```python
from build123d import *

# Parameters (mm, degrees)
F0_W            = 60
F0_H            = 55
F1_DEPTH        = 55
F2_T            = -3.5
F4_DEPTH        = 5
F6_D            = 3
F6_DEPTH        = 12
F6_TIP          = 0.9012909285
F8_D            = 3
F8_DEPTH        = 12
F8_TIP          = 0.9012909285
F7_W            = 41
F7_H            = 35
F9_DEPTH        = 25
F10_R           = 5
F11_DEPTH       = 7
F13_D           = 3
F13_DEPTH       = 5
F13_TIP         = 0.9012909285
F14_W           = 7
F14_H           = 3
F15_DEPTH       = 5
F16_W           = 7
F16_H           = 5
F17_DEPTH       = 5
F18_W           = 24
F18_H           = 6
F19_DEPTH       = 4
F21_D           = 3
F21_DEPTH       = 5
F21_TIP         = 0.9012909285
F23_D           = 3
F23_DEPTH       = 5
F23_TIP         = 0.9012909285
F24_W           = 10
F24_H           = 3
F25_DEPTH       = 10
F27_D           = 3.3
F27_DEPTH       = 5
F27_CSINK_D     = 6.72
F27_CSINK_ANGLE = 90
F27_TIP         = 0.9914200214
F29_D           = 3.3
F29_DEPTH       = 5
F29_CSINK_D     = 6.72
F29_CSINK_ANGLE = 90
F29_TIP         = 0.9914200214
F30_W           = 10
F30_H           = 3
F31_DEPTH       = 10
F32_DEPTH       = 10
F34_D           = 3.3
F34_DEPTH       = 5
F34_CSINK_D     = 6.72
F34_CSINK_ANGLE = 90
F34_TIP         = 0.9914200214


with BuildPart() as f1:
    # F0 (on Top) → F1 (new body)
    with BuildSketch(Plane.XY):
        Rectangle(F0_W, F0_H)
    extrude(amount=F1_DEPTH)

    # F2
    f2_openings = [f1.faces().sort_by_distance(p)[0] for p in [
        (0, 0, 55),
    ]]
    offset(amount=F2_T, openings=f2_openings)

    # F3 (on face) → F4 (cut)
    with BuildSketch(Plane.XZ.offset(27.5)):
        Polygon((19.05, 39.8), (-19.05, 39.8), (-19.05, 15.2), (0, 15.2), (19.05, 15.2), align=None)
    extrude(amount=-F4_DEPTH, mode=Mode.SUBTRACT)

    # F6
    with Locations(Plane.XZ.offset(27.5)):
        with Locations((-21.8598913223, 37.825), (-21.8598913223, 17.175), (21.5401086777, 17.175), (21.5401086777, 37.825)):
            Hole(F6_D / 2, depth=F6_DEPTH)
            with Locations((0, 0, -(F6_DEPTH + F6_TIP / 2))):  # 118° drill point
                Cone(0, F6_D / 2, F6_TIP, mode=Mode.SUBTRACT)

    # F8
    with Locations(Plane(origin=(-30, 0, 0), x_dir=(0, -1, 0), z_dir=(-1, 0, 0))):
        with Locations((-20, 47.5), (-20, 7.5), (20, 7.5), (20, 47.5)):
            Hole(F8_D / 2, depth=F8_DEPTH)
            with Locations((0, 0, -(F8_DEPTH + F8_TIP / 2))):  # 118° drill point
                Cone(0, F8_D / 2, F8_TIP, mode=Mode.SUBTRACT)

    # F7 (on face) → F9 (cut)
    with BuildSketch(Plane(origin=(-30, 0, 0), x_dir=(0, -1, 0), z_dir=(-1, 0, 0))):
        with Locations((0, 27.5)):
            Rectangle(F7_W, F7_H)
    extrude(amount=-F9_DEPTH, mode=Mode.SUBTRACT)

    # F10 (on face) → F11 (join)
    with BuildSketch(Plane.XY.offset(3.5)):
        with Locations((-17.7631583065, 0)):
            Circle(F10_R)
        with Locations((0, 15.3929423541)):
            Circle(F10_R)
        with Locations((16.9736854732, 0)):
            Circle(F10_R)
        with Locations((0, -14.607058838)):
            Circle(F10_R)
    extrude(amount=F11_DEPTH)

    # F13
    with Locations(Plane.XY.offset(10.5)):
        with Locations((0, 15.4706398025), (-17.7631583065, 0), (0, -14.2931165174), (17.22384803, 0)):
            Hole(F13_D / 2, depth=F13_DEPTH)
            with Locations((0, 0, -(F13_DEPTH + F13_TIP / 2))):  # 118° drill point
                Cone(0, F13_D / 2, F13_TIP, mode=Mode.SUBTRACT)

    # F14 (on face) → F15 (cut)
    with BuildSketch(Plane.YZ.offset(30)):
        with Locations((0, 28.8139954209)):
            Rectangle(F14_W, F14_H)
    extrude(amount=-F15_DEPTH, mode=Mode.SUBTRACT)

    # F16 (on face) → F17 (cut)
    with BuildSketch(Plane(origin=(0, 27.5, 0), x_dir=(-1, 0, 0), z_dir=(0, 1, 0))):
        with Locations((0, 29.2087327689)):
            Rectangle(F16_W, F16_H)
    extrude(amount=-F17_DEPTH, mode=Mode.SUBTRACT)

    # F18 (on face) → F19 (cut)
    with BuildSketch(Plane(origin=(-30, 0, 0), x_dir=(0, -1, 0), z_dir=(-1, 0, 0))):
        with Locations((0, 7)):
            Rectangle(F18_W, F18_H)
    extrude(amount=-F19_DEPTH, mode=Mode.SUBTRACT)

    # F21
    with Locations(Plane.YZ.offset(30)):
        with Locations((0, 43.075658381), (0, 14.3585540354)):
            Hole(F21_D / 2, depth=F21_DEPTH)
            with Locations((0, 0, -(F21_DEPTH + F21_TIP / 2))):  # 118° drill point
                Cone(0, F21_D / 2, F21_TIP, mode=Mode.SUBTRACT)

    # F23
    with Locations(Plane(origin=(0, 27.5, 0), x_dir=(-1, 0, 0), z_dir=(0, 1, 0))):
        with Locations((0, 37.1811050391), (0, 13.7660141307)):
            Hole(F23_D / 2, depth=F23_DEPTH)
            with Locations((0, 0, -(F23_DEPTH + F23_TIP / 2))):  # 118° drill point
                Cone(0, F23_D / 2, F23_TIP, mode=Mode.SUBTRACT)

    # F24 (on face) → F25 (join)
    with BuildSketch(Plane(origin=(0, 27.5, 0), x_dir=(-1, 0, 0), z_dir=(0, 1, 0))):
        with Locations((-25, 1.5)):
            Rectangle(F24_W, F24_H)
        with Locations((25, 1.5)):
            Rectangle(F24_W, F24_H)
    extrude(amount=F25_DEPTH)

    # F27
    with Locations(Plane.XY.offset(3)):
        with Locations((25, 32.5)):
            CounterSinkHole(F27_D / 2, F27_CSINK_D / 2, depth=F27_DEPTH, counter_sink_angle=F27_CSINK_ANGLE)
            with Locations((0, 0, -(F27_DEPTH + F27_TIP / 2))):  # 118° drill point
                Cone(0, F27_D / 2, F27_TIP, mode=Mode.SUBTRACT)

    # F29
    with Locations(Plane.XY.offset(3)):
        with Locations((-25, 32.5)):
            CounterSinkHole(F29_D / 2, F29_CSINK_D / 2, depth=F29_DEPTH, counter_sink_angle=F29_CSINK_ANGLE)
            with Locations((0, 0, -(F29_DEPTH + F29_TIP / 2))):  # 118° drill point
                Cone(0, F29_D / 2, F29_TIP, mode=Mode.SUBTRACT)

    # F30 (on face) → F31 (join)
    with BuildSketch(Plane.XZ.offset(27.5)):
        with Locations((-25, 1.5)):
            Rectangle(F30_W, F30_H)
    extrude(amount=F31_DEPTH)

    # F30 (on face) → F32 (join)
    with BuildSketch(Plane.XZ.offset(27.5)):
        with Locations((25, 1.5)):
            Rectangle(F30_W, F30_H)
    extrude(amount=F32_DEPTH)

    # F34
    with Locations(Plane.XY.offset(3)):
        with Locations((-25, -32.5), (25, -32.5)):
            CounterSinkHole(F34_D / 2, F34_CSINK_D / 2, depth=F34_DEPTH, counter_sink_angle=F34_CSINK_ANGLE)
            with Locations((0, 0, -(F34_DEPTH + F34_TIP / 2))):  # 118° drill point
                Cone(0, F34_D / 2, F34_TIP, mode=Mode.SUBTRACT)


solid = f1.part
```
Model file for the job. Use its own axes, mm. A direction names the side the tool comes from. Give positions to 0.01 mm unless a question says otherwise; leave off trailing zeros. Loops run counter-clockwise (first coordinate to the right, second up) from the corner with the lowest first, then second, coordinate; pieces in that order, holes last. Notation, with made-up numbers: (49, 45.25) -> (57, 45.25) arc R14 cw to (57, 67.25) -> close; hole circle Ø8 at (37.5, 12). An arc over 180 degrees is marked (long way). Use CSV: the item, a comma, the result in double quotes. Start each with the question number.
1) Slice it at B-B on x = 25. Give the cut face in (y, z).
2) Mould opens along Y. For faces 1 (the flat face through (25, -37.5, 2)), 2 (the cylindrical face through (-22.552, -25.726, 15.844)), 3 (the flat face through (1, -16, 10.5)), 4 (the flat face through (25, 37.5, 2)) say: released by +Y, released by -Y, zero draft, split by the parting line, or undercut.
3) Slice it at A-A on z = 34.5. Give the cut face in (x, y), plus the area to 3 significant figures.
4) Slice it at C-C on y = -17. Give the cut face in (x, z).
5) Slice it at D-D on x = 6. Give the cut face in (y, z), plus the area to 3 significant figures.
6) Flat gauge pins, fed straight in: pin 1 Ø8 at (x, y) = (9.5, -11) entering from -Z; pin 2 Ø24 at (y, z) = (-7, 27) entering from -X; pin 3 Ø0.9 at (x, z) = (28, 29) entering from -Y; pin 4 Ø4 at (x, z) = (0, 37.18) entering from -Y. Where does each tip first touch, or does it go through?
7) Tool access for faces 5 (the flat face through (-28, 16, 10)), 6 (the flat face through (19.05, -26, 27)), 7 (the cylindrical face through (-16.265, 0.066, 7.965)): list every direction of +Z, -Z, +X, -X, +Y, -Y with a clear straight run to the whole face (end or side of a thin tool).
8) Wall check: line 1 (Z direction, x = 0, y = 25.15); line 2 (Y direction, x = 0, z = 8.55); line 3 (Z direction, x = 13.5, y = -27). Give the ranges that are in metal, low to high.
Computed values:
1,outline,"(-37.5, 0) -> (-34.15, 0) -> (-34.15, 1.29) -> (-35.86, 3) -> (-37.5, 3) -> close; (-30.85, 0) -> (30.85, 0) -> (30.85, 1.29) -> (29.14, 3) -> (27.5, 3) -> (27.5, 55) -> (24, 55) -> (24, 3.5) -> (-24, 3.5) -> (-24, 55) -> (-27.5, 55) -> (-27.5, 3) -> (-29.14, 3) -> (-30.85, 1.29) -> close; (34.15, 0) -> (37.5, 0) -> (37.5, 3) -> (35.86, 3) -> (34.15, 1.29) -> close"
2,face 1,"released by -Y"
2,face 2,"zero draft"
2,face 3,"undercut"
2,face 4,"released by +Y"
3,outline,"(-30, -27.5) -> (-19.05, -27.5) -> (-19.05, -24) -> (-26.5, -24) -> (-26.5, -20.5) -> (-30, -20.5) -> close; (-30, 20.5) -> (-26.5, 20.5) -> (-26.5, 24) -> (26.5, 24) -> (26.5, -24) -> (19.05, -24) -> (19.05, -27.5) -> (30, -27.5) -> (30, 27.5) -> (-30, 27.5) -> close"
3,area,"479 mm^2"
4,outline,"(-30, 0) -> (30, 0) -> (30, 55) -> (26.5, 55) -> (26.5, 3.5) -> (4.39, 3.5) -> (4.39, 10.5) -> (-4.39, 10.5) -> (-4.39, 3.5) -> (-26.5, 3.5) -> (-26.5, 10) -> (-30, 10) -> close; (-30, 45) -> (-26.5, 45) -> (-26.5, 55) -> (-30, 55) -> close"
5,outline,"(-27.5, 0) -> (27.5, 0) -> (27.5, 55) -> (24, 55) -> (24, 3.5) -> (-24, 3.5) -> (-24, 15.2) -> (-27.5, 15.2) -> close; (-27.5, 39.8) -> (-24, 39.8) -> (-24, 55) -> (-27.5, 55) -> close"
5,area,"467 mm^2"
6,pin 1,"stops at z = 0"
6,pin 2,"stops at x = 26.5"
6,pin 3,"stops at y = -27.5"
6,pin 4,"stops at y = 24"
7,face 5,"-X"
7,face 6,"-Y"
7,face 7,"+Z"
8,line 1,"z = 0 to 12.27, 15.27 to 26.71, 31.71 to 35.68, 38.68 to 55"
8,line 2,"y = -27.5 to -24, -19.61 to -15.79, -12.79 to -9.61, 10.39 to 13.97, 16.97 to 20.39, 24 to 27.5"
8,line 3,"z = 0 to 15.2, 39.8 to 55"
